```python
from build123d import *

# Parameters (mm, degrees)
F0_R          = 1.5875
F1_DEPTH      = 6.35
F3_D          = 2.2606
F4_R          = 3.17499
F5_R          = 1.5875
F6_DEPTH      = 1.397
F7_R          = 1.5875
F8_DEPTH      = 1.397
F10_DEPTH     = 55.922402023
F11_W         = 0.635
F11_H         = 38.4961159321
F12_DEPTH     = 55.922402023
F13_T4_DEPTH  = 12.6181992369
F13_T9_DEPTH  = 12.6181992369
F13_T14_DEPTH = 11.9054737587
F13_T19_DEPTH = 11.9054737587
F15_DEPTH     = 1.27
F17_DEPTH     = 1.27


# Not quite as in the source:
# - a fillet or chamfer that OpenCascade refuses, or shapes differently, is made with other operations: its cross-section is extruded or revolved along the edge and cut away or added
# - a fillet or chamfer is up to 0.001 mm smaller than in the source, because OpenCascade refuses the exact size


with BuildPart() as f1:
    # F0 (on Front) → F1 (new body)
    with BuildSketch(Plane.XZ):
        with BuildLine():
            Line((6.6774413169, -0.1881909028), (30.734, -0.1881909028))
            Line((30.734, -0.1881909028), (30.734, 3.8758090972))
            Line((30.734, 3.8758090972), (24.638, 3.8758090972))
            Line((24.638, 3.8758090972), (24.638, 5.3998090972))
            Line((24.638, 5.3998090972), (0.8976435847, 5.3998090972))
            ThreePointArc((0.8976435847, 5.3998090972), (-1.8031521678, 4.7037868469), (-3.8311440773, 2.7891084184))
            Line((-3.8311440773, 2.7891084184), (-32.4066881959, -42.5968826722))
            ThreePointArc((-32.4066881959, -42.5968826722), (-31.4949255527, -46.7722351265), (-27.3046829217, -45.931553303))
            Line((-27.3046829217, -45.931553303), (2.052552643, -2.6399274008))
            ThreePointArc((2.052552643, -2.6399274008), (4.0601618562, -0.8390265117), (6.6774413169, -0.1881909028))
        make_face()
        with Locations((-29.8273494711, -44.2208641201)):
            Circle(F0_R, mode=Mode.SUBTRACT)
        Circle(F0_R, mode=Mode.SUBTRACT)
    extrude(amount=F1_DEPTH)

    # F3 (through all)
    with Locations(Plane.XY.offset(3.8758090972)):
        with Locations((27.686, -3.175)):
            Hole(F3_D / 2)

    # F4 (radius 3.175 in the source; OpenCascade refuses exactly that, so slightly less here)
    f4_edges = [f1.edges().sort_by_distance(p)[0] for p in [
        (30.734, -6.35, 1.843809),
        (30.734, 0, 1.843809),
    ]]
    fillet(f4_edges, radius=F4_R)

    # F5 (on face) → F6 (join)
    with BuildSketch(Plane.XZ.offset(6.35)):
        with BuildLine():
            Line((-27.3046829217, -45.931553303), (-22.3122897877, -38.5695244281))
            Line((-22.3122897877, -38.5695244281), (-27.7252582931, -35.1614569468))
            Line((-27.7252582931, -35.1614569468), (-32.4066881959, -42.5968826722))
            ThreePointArc((-32.4066881959, -42.5968826722), (-31.4949255527, -46.7722351265), (-27.3046829217, -45.931553303))
        make_face()
        with Locations((-29.8273494711, -44.2208641201)):
            Circle(F5_R, mode=Mode.SUBTRACT)
    extrude(amount=F6_DEPTH)

    # F7 (on face) → F8 (join)
    with BuildSketch(Plane(origin=(0, 0, 0), x_dir=(-1, 0, 0), z_dir=(0, 1, 0))):
        with BuildLine():
            ThreePointArc((27.3046829217, -45.931553303), (31.4949255527, -46.7722351265), (32.4066881959, -42.5968826722))
            Line((32.4066881959, -42.5968826722), (27.7252582931, -35.1614569468))
            Line((27.7252582931, -35.1614569468), (22.3122897877, -38.5695244281))
            Line((22.3122897877, -38.5695244281), (27.3046829217, -45.931553303))
        make_face()
        with Locations((29.8273494711, -44.2208641201)):
            Circle(F7_R, mode=Mode.SUBTRACT)
    extrude(amount=F8_DEPTH)

    # F9 (on face) → F10 (cut, through all)
    with BuildSketch(Plane(origin=(-4.0011143857, 0, 2.519147823), x_dir=(0, -1, 0), z_dir=(-0.8462397391, 0, 0.5328023123))):
        with BuildLine():
            Line((1.524, -56.3615332831), (4.826, -56.3615332831))
            Line((4.826, -56.3615332831), (4.826, -46.0745332831))
            ThreePointArc((4.826, -46.0745332831), (3.175, -44.4235332831), (1.524, -46.0745332831))
            Line((1.524, -46.0745332831), (1.524, -56.3615332831))
        make_face()
    extrude(amount=-F10_DEPTH, mode=Mode.SUBTRACT)

    # F11 (on face) → F12 (cut, through all)
    with BuildSketch(Plane(origin=(-4.0011143857, 0, 2.519147823), x_dir=(0, -1, 0), z_dir=(-0.8462397391, 0, 0.5328023123))):
        with Locations((0.3175, -25.2790459142)):
            Rectangle(F11_W, F11_H)
        with Locations((6.0325, -25.2790459142)):
            Rectangle(F11_W, F11_H)
    extrude(amount=-F12_DEPTH, mode=Mode.SUBTRACT)

    # F13: fillet of radius 2.54 on 4 edges, made by hand


with BuildPart() as f13_tool2:
    # F13_s3 → F13_t4 (new body)
    with BuildSketch(Plane(origin=(-4.0011143857, 0, 2.519147823), x_dir=(0, 1, 0), z_dir=(0.8462397391, 0, -0.5328023123))):
        with BuildLine():
            ThreePointArc((-7.747, -44.5271038802), (-6.2875244601, -43.6448593529), (-5.715, -42.0384223016))
            Line((-5.715, -42.0384223016), (-5.715, -44.5271038802))
            Line((-5.715, -44.5271038802), (-7.747, -44.5271038802))
        make_face()
    extrude(amount=F13_T4_DEPTH)

    split(bisect_by=Plane(origin=(2.6322854892, 0, -1.7850247841), x_dir=(0, 1, 0), z_dir=(-0.8276465057, 0, 0.5612497319)), keep=Keep.TOP)


with BuildPart() as f1_1:
    add(f1.part)

    # F13_t1: union F13_tool2
    add(f13_tool2.part)


with BuildPart() as f13_tool7:
    # F13_s8 → F13_t9 (new body)
    with BuildSketch(Plane(origin=(-4.0011143857, 0, 2.519147823), x_dir=(0, 1, 0), z_dir=(0.8462397391, 0, -0.5328023123))):
        with BuildLine():
            ThreePointArc((-0.635, -42.0384223016), (-0.0624755399, -43.6448593529), (1.397, -44.5271038802))
            Line((1.397, -44.5271038802), (-0.635, -44.5271038802))
            Line((-0.635, -44.5271038802), (-0.635, -42.0384223016))
        make_face()
    extrude(amount=F13_T9_DEPTH)

    split(bisect_by=Plane(origin=(2.6322854892, 0, -1.7850247841), x_dir=(0, 1, 0), z_dir=(-0.8276465057, 0, 0.5612497319)), keep=Keep.TOP)


with BuildPart() as f1_2:
    add(f1_1.part)

    # F13_t6: union F13_tool7
    add(f13_tool7.part)


with BuildPart() as f13_tool12:
    # F13_s13 → F13_t14 (new body)
    with BuildSketch(Plane(origin=(-4.0011143857, 0, 2.519147823), x_dir=(0, 1, 0), z_dir=(0.8462397391, 0, -0.5328023123))):
        with BuildLine():
            ThreePointArc((0, -6.0309879482), (-0.4709524406, -6.8130144186), (-0.635, -7.7110400307))
            Line((-0.635, -7.7110400307), (-0.635, -6.0309879482))
            Line((-0.635, -6.0309879482), (0, -6.0309879482))
        make_face()
    extrude(amount=F13_T14_DEPTH)

    split(bisect_by=Plane(origin=(2.6322854892, 0, -1.7850247841), x_dir=(0, 1, 0), z_dir=(-0.8276465057, 0, 0.5612497319)), keep=Keep.TOP)


with BuildPart() as f1_3:
    add(f1_2.part)

    # F13_t11: union F13_tool12
    add(f13_tool12.part)


with BuildPart() as f13_tool17:
    # F13_s18 → F13_t19 (new body)
    with BuildSketch(Plane(origin=(-4.0011143857, 0, 2.519147823), x_dir=(0, 1, 0), z_dir=(0.8462397391, 0, -0.5328023123))):
        with BuildLine():
            ThreePointArc((-5.715, -7.7110400307), (-5.8790475594, -6.8130144186), (-6.35, -6.0309879482))
            Line((-6.35, -6.0309879482), (-5.715, -6.0309879482))
            Line((-5.715, -6.0309879482), (-5.715, -7.7110400307))
        make_face()
    extrude(amount=F13_T19_DEPTH)

    split(bisect_by=Plane(origin=(2.6322854892, 0, -1.7850247841), x_dir=(0, 1, 0), z_dir=(-0.8276465057, 0, 0.5612497319)), keep=Keep.TOP)


with BuildPart() as f1_4:
    add(f1_3.part)

    # F13_t16: union F13_tool17
    add(f13_tool17.part)

    # F14 (on face) → F15 (cut)
    with BuildSketch(Plane.XZ.offset(5.715)):
        with BuildLine():
            ThreePointArc((-22.5785911234, -29.4180135738), (-22.8665153513, -30.9463544712), (-21.9894083128, -32.2306478578))
            ThreePointArc((-21.9894083128, -32.2306478578), (-20.4610674153, -32.5185720857), (-19.1767740287, -31.6414650472))
            Line((-19.1767740287, -31.6414650472), (-5.9518651728, -11.4077331396))
            ThreePointArc((-5.9518651728, -11.4077331396), (-5.6639409449, -9.8793922421), (-6.5410479835, -8.5950988555))
            ThreePointArc((-6.5410479835, -8.5950988555), (-8.0693888809, -8.3071746276), (-9.3536822675, -9.1842816662))
            Line((-9.3536822675, -9.1842816662), (-22.5785911234, -29.4180135738))
        make_face()
    extrude(amount=-F15_DEPTH, mode=Mode.SUBTRACT)

    # F16 (on face) → F17 (cut)
    with BuildSketch(Plane(origin=(0, -0.635, 0), x_dir=(-1, 0, 0), z_dir=(0, 1, 0))):
        with BuildLine():
            ThreePointArc((19.1767740287, -31.6414650472), (21.9894083128, -32.2306478578), (22.5785911234, -29.4180135738))
            Line((22.5785911234, -29.4180135738), (9.3536822675, -9.1842816662))
            ThreePointArc((9.3536822675, -9.1842816662), (6.5410479835, -8.5950988555), (5.9518651728, -11.4077331396))
            Line((5.9518651728, -11.4077331396), (19.1767740287, -31.6414650472))
        make_face()
    extrude(amount=-F17_DEPTH, mode=Mode.SUBTRACT)


solid = f1_4.part
```
Geometry: final body of the model. Coordinates: model frame, mm. A direction names the side the tool comes from. Coordinates: 2 decimals unless noted, no trailing zeros. Write each loop counter-clockwise with the first axis right and the second up, starting at its lowest first coordinate (ties: lowest second). Pieces come first, ordered by that corner, then holes. Notation, with made-up numbers: M 28,45.5 L 58,45.5 A21 ccw 58,80.5 Z; hole C 17.25,73 d10. An arc over 180 degrees is marked long. Use CSV: the item, a comma, the result in double quotes. Start each with the question number.
1. Cut plane C-C on x = -17. Return the cut outline in (y, z) (3 decimals), plus the area to 3 significant figures.
2. Cut plane B-B on z = -27.5. Return the cut outline in (x, y) (3 decimals).
3. Ray query, probe 1 along Z at (x, y) = (-11, -5.5); probe 2 along Y at (x, z) = (-23, -34.5) (3 decimals); probe 3 along X at (y, z) = (-4.75, -17). Return the intervals inside material, ascending.
4. Mould query, pull axis Z, two halves, no side actions, for faces 6 (the face through (-31.439, -0.084, -46.808)), 7 (the face through (-30.034, -6.266, -42.647)), 8 (the face through (24.638, -3, 5)). Classes: pulls with the +Z half, pulls with the -Z half, needs draft (parallel to the pull), parting line crosses it, or undercut.
5. Cut plane D-D on x = 7.5. Return the cut outline in (y, z), plus the area to 3 significant figures.
6. First-contact query: P1, Ø12, axis at x = -15.5, z = -15.5, coming from the -Y side (3 decimals); P2, Ø5, axis at x = -2.5, z = -8, coming from the -Y side; P3, Ø6, axis at x = -14.5, z = -20.5, coming from the +Y side (3 decimals); P4, Ø1.8, axis at x = 27.686, y = -3.175, coming from the +Z side. Flat tips, straight axial feed; report the tip coordinate or a pass-through.
7. Reachability of faces 1 (the face through (-14, -1.905, -20)), 2 (the face through (26, -3, 3.876)), 3 (the face through (-12.66, -5.09, -21.67)), 4 (the face through (-24.56, -6.3, -36.13)), 5 (the face through (-28, 1.397, -41)) from +Z, -Z, +X, -X, +Y, -Y: full face, straight path, thin tool, end or side. Return the list, or none.
8. Cut plane A-A on x = 0. Return the cut outline in (y, z).
Entries:
1,outline,"M -5.715,-30.736 L -0.635,-30.736 L -0.635,-28.311 L -1.905,-28.311 L -1.905,-20.883 L -0.635,-20.883 L -0.635,-18.127 L -5.715,-18.127 L -5.715,-20.883 L -4.445,-20.883 L -4.445,-28.311 L -5.715,-28.311 Z"
1,area,"45.2 mm²"
2,outline,"M -22.902,-5.715 L -21.325,-5.715 L -21.325,-4.445 L -16.47,-4.445 L -16.47,-5.715 L -14.806,-5.715 L -14.806,-0.635 L -16.47,-0.635 L -16.47,-1.905 L -21.325,-1.905 L -21.325,-0.635 L -22.902,-0.635 Z"
3,probe 1,"-21.89 to -19.13, -11.7 to -8.6"
3,probe 2,"-5.715 to -0.635"
3,probe 3,"-16.29 to -14.46, -9.61 to -7.69"
4,face 6,"parting line crosses it"
4,face 7,"undercut"
4,face 8,"needs draft"
5,outline,"M -6.35,-0.19 L 0,-0.19 L 0,5.4 L -6.35,5.4 Z"
5,area,"35.5 mm²"
6,P1,"y = -5.715"
6,P2,"y = -6.35"
6,P3,"y = -0.635"
6,P4,"through"
7,face 1,"+Y"
7,face 2,"+Z, +X, +Y, -Y"
7,face 3,"-Y"
7,face 4,"+Z, +X, -Y"
7,face 5,"+Z, -Z, +X, -X, +Y"
8,outline,"M -6.35,-5.67 L 0,-5.67 L 0,-1.59 L -6.35,-1.59 Z; M -6.35,1.59 L 0,1.59 L 0,5.33 L -6.35,5.33 Z"
